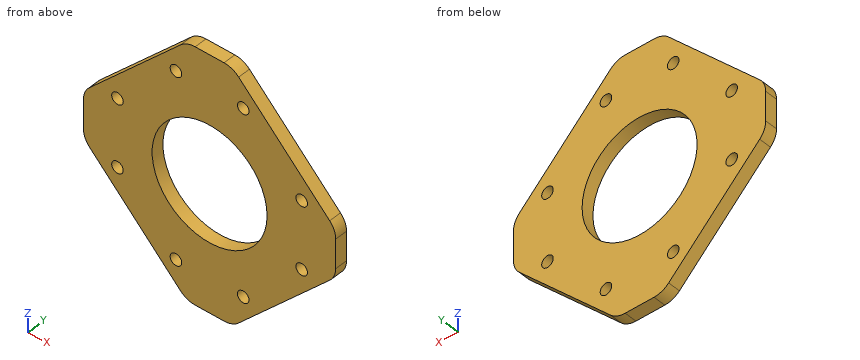
```python
from build123d import *

# Parameters (mm, degrees)
SKETCH1_R           = 13.9
SKETCH1_R_2         = 1.4
BOSS_EXTRUDE1_DEPTH = 3


with BuildPart() as part:
    # Sketch1 → Boss-Extrude1 (new body)
    with BuildSketch(Plane(origin=(0, 0, 0), x_dir=(1, 0, 0), z_dir=(0, 1, 0))):
        with BuildLine():
            Line((3.491378029, 30.5), (-3.491378029, 30.5))
            ThreePointArc((-3.491378029, 30.5), (-5.40479519, 30.119397663), (-7.026911935, 29.035533906))
            Line((-7.026911935, 29.035533906), (-29.035533906, 7.026911935))
            ThreePointArc((-29.035533906, 7.026911935), (-30.119397663, 5.40479519), (-30.5, 3.491378029))
            Line((-30.5, 3.491378029), (-30.5, -3.491378029))
            ThreePointArc((-30.5, -3.491378029), (-30.119397663, -5.40479519), (-29.035533906, -7.026911935))
            Line((-29.035533906, -7.026911935), (-7.026911935, -29.035533906))
            ThreePointArc((-7.026911935, -29.035533906), (-5.40479519, -30.119397663), (-3.491378029, -30.5))
            Line((-3.491378029, -30.5), (3.491378029, -30.5))
            ThreePointArc((3.491378029, -30.5), (5.40479519, -30.119397663), (7.026911935, -29.035533906))
            Line((7.026911935, -29.035533906), (29.035533906, -7.026911935))
            ThreePointArc((29.035533906, -7.026911935), (30.119397663, -5.40479519), (30.5, -3.491378029))
            Line((30.5, -3.491378029), (30.5, 3.491378029))
            ThreePointArc((30.5, 3.491378029), (30.119397663, 5.40479519), (29.035533906, 7.026911935))
            Line((29.035533906, 7.026911935), (7.026911935, 29.035533906))
            ThreePointArc((7.026911935, 29.035533906), (5.40479519, 30.119397663), (3.491378029, 30.5))
        make_face()
        Circle(SKETCH1_R, mode=Mode.SUBTRACT)
        with Locations((8.131727984, -22.273863607)):
            Circle(SKETCH1_R_2, mode=Mode.SUBTRACT)
        with Locations((-8.131727984, -22.273863607)):
            Circle(SKETCH1_R_2, mode=Mode.SUBTRACT)
        with Locations((-22.273863607, -8.131727984)):
            Circle(SKETCH1_R_2, mode=Mode.SUBTRACT)
        with Locations((22.273863607, -8.131727984)):
            Circle(SKETCH1_R_2, mode=Mode.SUBTRACT)
        with Locations((22.273863607, 8.131727984)):
            Circle(SKETCH1_R_2, mode=Mode.SUBTRACT)
        with Locations((8.131727984, 22.273863607)):
            Circle(SKETCH1_R_2, mode=Mode.SUBTRACT)
        with Locations((-8.131727984, 22.273863607)):
            Circle(SKETCH1_R_2, mode=Mode.SUBTRACT)
        with Locations((-22.273863607, 8.131727984)):
            Circle(SKETCH1_R_2, mode=Mode.SUBTRACT)
    extrude(amount=BOSS_EXTRUDE1_DEPTH)


solid = part.part
```
Model file for the job. Use its own axes, mm. Give positions to 0.01 mm unless a question says otherwise; leave off trailing zeros. Loops run counter-clockwise (first coordinate to the right, second up) from the corner with the lowest first, then second, coordinate; pieces in that order, holes last. Notation, with made-up numbers: (-26, -29.5) - (27, -29.5) arc R24 ccw to (27, -9.5) - close; hole circle Ø4 at (-22.5, 56). An arc over 180 degrees is marked (long way). One line per item, written item: value. Start each with the question number.
1. Pin check, flat tips, straight feed: pin 1 (2.5 mm diameter, centred on x = 22.27, z = 8.13, fed in from -Y); pin 2 (1 mm diameter, centred on y = 1.5, z = -10.5, fed in from +X). Stop position of each tip, or through.
2. Probe L1, parallel to Z at x = 23.5, y = 2.55; L2, parallel to Z at x = 21, y = 1.8; L3, parallel to X at y = 1.8, z = -7.5. List the from-to ranges inside material, lowest first. Write a range as from..to.
3. Slice it at A-A (z = 0). List the corners of the cut face in (x, y), plus the area to 3 significant figures.
4. Slice it at C-C (y = 0.75). Give the number of separate pieces and of enclosed holes in the cut face, plus the area to 3 significant figures.
5. Slice it at D-D (z = -17). List the corners of the cut face in (x, y), plus the area to 3 significant figures.
6. Slice it at B-B (x = 0). List the corners of the cut face in (y, z).
Solution:
1. pin 1: passes through
1. pin 2: stops at x = 26.06
2. L1: z = -12.56..-8.81, -7.46..7.46, 8.81..12.56
2. L2: z = -15.06..-8.71, -7.55..7.55, 8.71..15.06
2. L3: x = -28.56..-23.52, -21.02..-11.7, 11.7..21.02, 23.52..28.56
3. outline: (-30.5, 0) - (-13.9, 0) - (-13.9, 3) - (-30.5, 3) - close; (13.9, 0) - (30.5, 0) - (30.5, 3) - (13.9, 3) - close
3. area: 99.6 mm^2
4. separate pieces: 1
4. enclosed holes: 9
4. area: 1,820 mm^2
5. outline: (-19.06, 0) - (19.06, 0) - (19.06, 3) - (-19.06, 3) - close
5. area: 114 mm^2
6. outline: (0, -30.5) - (3, -30.5) - (3, -13.9) - (0, -13.9) - close; (0, 13.9) - (3, 13.9) - (3, 30.5) - (0, 30.5) - close
